Source: CAD feature listing. Evaluate the final solid. Frame: model axes, mm. Give positions to 0.01 mm unless a question says otherwise; leave off trailing zeros. Order: outer loops, then holes, each group sorted by start corner. A loop starts at its lowest first (then second) coordinate and runs counter-clockwise, first axis right, second up. Notation, with made-up numbers: (-34, 69) -> (6, 69) arc R12 cw to (6, 88) -> close; hole circle Ø8 at (26.5, 52). An arc over 180 degrees is marked (long way). Use one line per item in the form item = value. Start each with the question number.
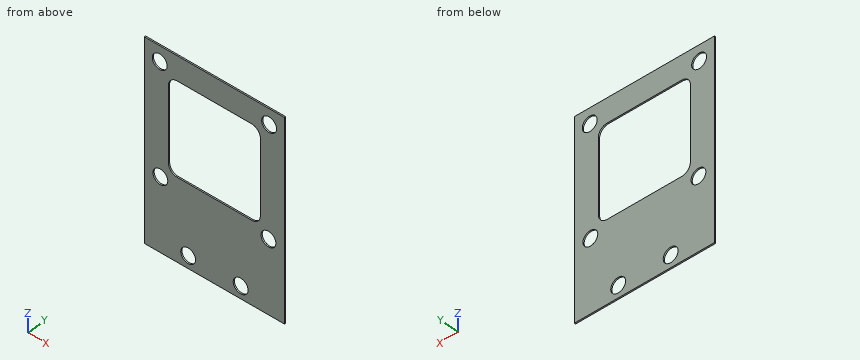
Autodesk Inventor part; units mm, degrees
ref_plane "YZ Plane" through (0, 0, 0) normal (1, 0, 0) x (0, 1, 0)
ref_plane "XZ Plane" through (0, 0, 0) normal (0, 1, 0) x (-1, 0, 0)
ref_plane "XY Plane" through (0, 0, 0) normal (0, 0, 1) x (1, 0, 0)
sketch "スケッチ1" plane through (0, 0, 0) normal (0, 1, 0) x (-1, 0, 0)
  line L0 (16, -31) -> (16, 14)
  line L1 (16, 14) -> (-16, 14)
  line L2 (-16, 14) -> (-16, -31)
  line L3 (-16, -31) -> (16, -31)
  line L4 (0, 0) -> (0, -32.6995) construction
  point P0 (0, 14)
  dimension "d0" = 45
  dimension "d1" = 32
  dimension "d2" = 14
extrude "押し出し1" add sketch "スケッチ1" along normal blind 0.3
sketch "スケッチ4" plane through (0, 0.3, 0) normal (0, 1, 0) x (1, 0, 0)
  line L0 (0, 0) -> (-18.7084, 0) construction
  circle A0 centre (-6, 28.2) radius 1.7
  circle A1 centre (6, 28.2) radius 1.7
  line L1 (0, 0) -> (0, 29.6633) construction
  line L2 (16, 31) -> (-16, 31)
  point P0 (0, 31)
  dimension "d35" = 3.4
  dimension "d36" = 3.4
  dimension "d37" = 6
  dimension "d38" = 2.8
extrude "押し出し3" cut sketch "スケッチ4" against normal through all
sketch "スケッチ7" plane through (0, 0.3, 0) normal (0, 1, 0) x (1, 0, 0)
  circle A0 centre (-12.5, -10.5) radius 1.7
  circle A1 centre (12.5, -10.5) radius 1.7
  circle A2 centre (12.3554, 14.5) radius 1.7
  circle A3 centre (-12.3554, 14.5) radius 1.7
  line L0 (0, 0) -> (0, 34.4459) construction
  point P0 (-16, -14)
  dimension "d47" = 3.4
  dimension "d48" = 3.4
  dimension "d49" = 3.4
  dimension "d50" = 3.4
  dimension "d51" = 25
  dimension "d52" = 25
  dimension "d55" = 3.5
extrude "押し出し6" cut sketch "スケッチ7" against normal through all
sketch "スケッチ8" plane through (0, 0.3, 0) normal (0, 1, 0) x (1, 0, 0)
  line L0 (-10.5, -8.5) -> (10.5, -8.5)
  line L1 (10.5, -8.5) -> (10.5, 12.5)
  line L2 (10.5, 12.5) -> (-10.5, 12.5)
  line L3 (-10.5, 12.5) -> (-10.5, -8.5)
  line L4 (0, 0) -> (0, 16.5634) construction
  point P0 (-16, -14)
  dimension "d56" = 21
  dimension "d57" = 21
  dimension "d58" = 5.5
extrude "押し出し7" cut sketch "スケッチ8" against normal through all
fillet "フィレット1" radius 2 4 edges at (-10.5, 0.15, -12.5) (-10.5, 0.15, 8.5) (10.5, 0.15, 8.5) (10.5, 0.15, -12.5)
properties part number "B_holder_middle_muti-holes" material "ステンレス鋼 440C"
1) Cut plane A-A, the plane y = 0.1. Return the cut outline in (x, z), plus the area to 3 significant figures.
2) Cut plane B-B, the plane x = 6. Return the cut outline in (y, z).
3) Cut plane C-C, the plane z = -9. Return the cut outline in (x, y).
4) Material intervals for probe 1 along Z at (x, y) = (12.5, 0.2); probe 2 along Z at (x, y) = (-6, 0.2); probe 3 along X at (y, z) = (0.15, 10.5), sorted ascending.
5) Cut plane D-D, the plane z = -14.5. Return the cut outline in (x, y).
Output values:
q1.outline = (-16, -31) -> (16, -31) -> (16, 14) -> (-16, 14) -> close; hole circle Ø3.4 at (-12.5, 10.5); hole circle Ø3.4 at (-12.36, -14.5); hole (-10.5, -10.5) arc R2 ccw to (-8.5, -12.5) -> (8.5, -12.5) arc R2 ccw to (10.5, -10.5) -> (10.5, 6.5) arc R2 ccw to (8.5, 8.5) -> (-8.5, 8.5) arc R2 ccw to (-10.5, 6.5) -> close; hole circle Ø3.4 at (-6, -28.2); hole circle Ø3.4 at (6, -28.2); hole circle Ø3.4 at (12.36, -14.5); hole circle Ø3.4 at (12.5, 10.5)
q1.area = 948 mm^2
q2.outline = (0, -31) -> (0.3, -31) -> (0.3, -29.9) -> (0, -29.9) -> close; (0, -26.5) -> (0.3, -26.5) -> (0.3, -12.5) -> (0, -12.5) -> close; (0, 8.5) -> (0.3, 8.5) -> (0.3, 14) -> (0, 14) -> close
q3.outline = (-16, 0) -> (-10.5, 0) -> (-10.5, 0.3) -> (-16, 0.3) -> close; (10.5, 0) -> (16, 0) -> (16, 0.3) -> (10.5, 0.3) -> close
q4.probe_1 = -31 to -16.19, -12.81 to 8.8, 12.2 to 14
q4.probe_2 = -31 to -29.9, -26.5 to -12.5, 8.5 to 14
q4.probe_3 = -16 to -14.2, -10.8 to 10.8, 14.2 to 16
q5.outline = (-16, 0) -> (-14.06, 0) -> (-14.06, 0.3) -> (-16, 0.3) -> close; (-10.66, 0) -> (10.66, 0) -> (10.66, 0.3) -> (-10.66, 0.3) -> close; (14.06, 0) -> (16, 0) -> (16, 0.3) -> (14.06, 0.3) -> close
